Here's how the part is built. I have some questions about the finished solid (model axes, mm). A direction names the side the tool comes from. Give positions to 0.01 mm unless a question says otherwise; leave off trailing zeros. Write each loop counter-clockwise with the first axis right and the second up, starting at its lowest first coordinate (ties: lowest second). Pieces come first, ordered by that corner, then holes. Notation, with made-up numbers: (32.25, 35.25) - (36.25, 35.25) arc R25 cw to (36.25, 60.25) - close; hole circle Ø7 at (54.25, -30). An arc over 180 degrees is marked (long way). One line per item, written item: value. Start each with the question number.
1) Imagine slicing it at A-A on x = 0. Write out the boundary of the cut face in (y, z), plus the area to 3 significant figures.
2) I'm going to push flat-ended pins straight in: P1, Ø1.5, axis at y = 0, z = 5, coming from the +X side; P2, Ø2, axis at x = -0.5, z = 3.5, coming from the -Y side; P3, Ø1.6, axis at x = 0, y = -0.5, coming from the -Z side. Where does each tip first touch, or does it pass through?
3) Imagine slicing it at B-B on z = -0.5. Write out the boundary of the cut face in (x, y).
4) Please list where these lines run through material, in increasing order: L1, parallel to Z at x = 0.9, y = -2.45; L2, parallel to Y at x = -0.9, z = 1; L3, parallel to Z at x = -1.1, y = 0.95. Write a range as [from, to].
5) On a 3-axis mill with a long thin cutter (end or side, diameter ignored), from which of +Z, -Z, +X, -X, +Y, -Y can I reach the whole of each face in a straight line? I mean faces 1 (the cylindrical face through (-2.86, -0.11, 0.3)), 2 (the cylindrical face through (-0.54, -2.44, 3.02)). Say none if no direction works.
6) Imagine slicing it at C-C on y = 0. Write out the boundary of the cut face in (x, z), plus the area to 3 significant figures.
7) Imagine slicing it at D-D on z = 2.5. Write out the boundary of the cut face in (x, y).
from build123d import *

# Parameters (mm, degrees)
EXTRUDE_1_DEPTH = 0.6
SKETCH_2_R      = 2.5
EXTRUDE_2_DEPTH = 7.4
FILLET_1_R      = 2.5
SKETCH_3_R      = 0.2
EXTRUDE_3_DEPTH = 3


with BuildPart() as part:
    # 草图1 → 凸台-拉伸1 (new body)
    with BuildSketch(Plane.XY):
        with BuildLine():
            Line((2.6, 1.2), (2.6, -1.2))
            ThreePointArc((2.6, -1.2), (-2.863564213, 0), (2.6, 1.2))
        make_face()
    extrude(amount=EXTRUDE_1_DEPTH)

    # 草图2 → 凸台-拉伸2 (add)
    with BuildSketch(Plane.XY.offset(0.6)):
        Circle(SKETCH_2_R)
    extrude(amount=EXTRUDE_2_DEPTH)

    # 圆角1
    fillet_1_edges = [part.edges().sort_by_distance(p)[0] for p in [
        (-2.5, 0, 8),
    ]]
    fillet(fillet_1_edges, radius=FILLET_1_R)

    # 草图3 → 凸台-拉伸3 (add)
    with BuildSketch(Plane(origin=(0, 0, 0), x_dir=(-1, 0, 0), z_dir=(0, 0, -1))):
        with Locations(Location((1.27, 0, 0), (0, 0, 180))):
            Circle(SKETCH_3_R)
        with Locations(Location((-1.27, 0, 0), (0, 0, 180))):
            Circle(SKETCH_3_R)
    extrude(amount=EXTRUDE_3_DEPTH)


solid = part.part
Numbers:
1. outline: (-2.86, 0) - (2.86, 0) - (2.86, 0.6) - (2.5, 0.6) - (2.5, 5.5) arc R2.5 ccw to (-2.5, 5.5) - (-2.5, 0.6) - (-2.86, 0.6) - close
1. area: 37.8 mm^2
2. P1: x = 2.5
2. P2: y = -2.5
2. P3: z = 0
3. outline: circle Ø0.4 at (-1.27, 0); circle Ø0.4 at (1.27, 0)
4. L1: [0, 0.6]
4. L2: [-2.33, 2.33]
4. L3: [0, 7.53]
5. face 1: +Z, -Z
5. face 2: +Z
6. outline: (-2.86, 0) - (-1.47, 0) - (-1.47, -3) - (-1.07, -3) - (-1.07, 0) - (1.07, 0) - (1.07, -3) - (1.47, -3) - (1.47, 0) - (2.6, 0) - (2.6, 0.6) - (2.5, 0.6) - (2.5, 5.5) arc R2.5 ccw to (-2.5, 5.5) - (-2.5, 0.6) - (-2.86, 0.6) - close
6. area: 40.0 mm^2
7. outline: circle Ø5 at (0, 0)
